For this review, use the dimensioned drawing (mm, ordinates from the lowest corner) and the shaded views. Coordinates: 2 decimals unless noted, no trailing zeros. Order: outer loops, then holes, each group sorted by start corner. A loop starts at its lowest first (then second) coordinate and runs counter-clockwise, first axis right, second up. Notation, with made-up numbers: M 38,16.5 L 52,16.5 A18 cw 52,27.5 Z; hole C 7,80.25 d4. An arc over 180 degrees is marked long. Answer in a Markdown table with one row per item.
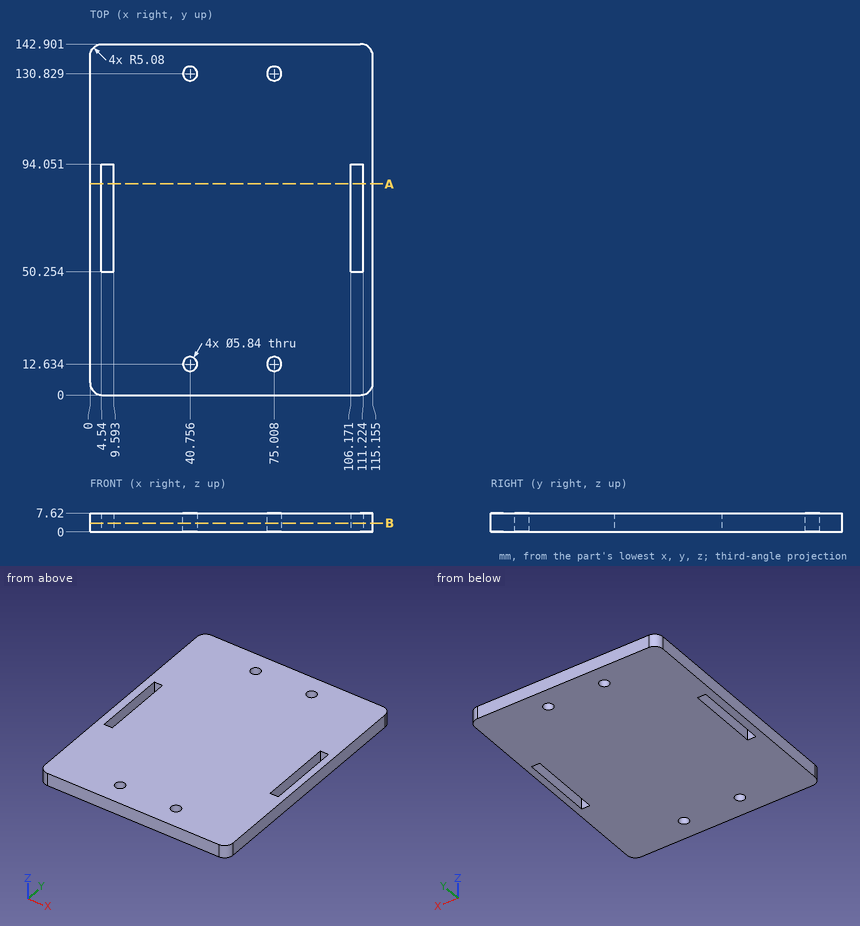
(1) Take a section at A-A (y = 86). Write out the cut boundary in (x, z) (1 decimal).
Report:
| item | result |
|---|---|
| outline | M 0,0 L 4.5,0 L 4.5,7.6 L 0,7.6 Z; M 9.6,0 L 106.2,0 L 106.2,7.6 L 9.6,7.6 Z; M 111.2,0 L 115.2,0 L 115.2,7.6 L 111.2,7.6 Z |
(2) To check wall thickness, follow line 1 (X direction, y = 72, z = 4) (1 decimal); line 2 (X direction, y = 12, z = 1.5) (1 decimal). State the ranges of each line that lie inside material, in increasing order. Write a range as [from, to].
Report:
| item | result |
|---|---|
| line 1 | [0, 4.5], [9.6, 106.2], [111.2, 115.2] |
| line 2 | [0, 37.9], [43.6, 72.2], [77.9, 115.2] |
(3) Take a section at B-B (z = 3.5). State how many separate pieces and enclosed holes the cut face has, then the cut area to 3 significant figures.
Report:
| item | result |
|---|---|
| separate pieces | 1 |
| enclosed holes | 6 |
| area | 15,900 mm^2 |
(4) Insertion check: P1, Ø5, axis at x = 15, y = 42.5, coming from the -Z side; P2, Ø5.5, axis at x = 75.01, y = 130.83, coming from the +Z side. Each pin has a flat end and moves straight along its axis. Give the tip position at first contact, or say it passes through.
Report:
| item | result |
|---|---|
| P1 | z = 0 |
| P2 | through |
